from build123d import *

# Parameters (mm, degrees)
F0_W     = 450
F0_H     = 200
F1_DEPTH = 20
F3_DEPTH = 450
F4_R     = 15
F5_DEPTH = 5
F4_R_2   = 32
F4_R_3   = 30.75
F6_DEPTH = 1
F4_R_4   = 5
F7_DEPTH = 30


with BuildPart() as f1:
    # F0 (on Top) → F1 (new body)
    with BuildSketch(Plane.XY):
        Rectangle(F0_W, F0_H)
    extrude(amount=F1_DEPTH)

    # F2 (on face) → F3 (join)
    with BuildSketch(Plane.YZ.offset(225)):
        Polygon((100, 37.4977327052), (-100, 20), (100, 20), align=None)
    extrude(amount=-F3_DEPTH)

    # F4 (on face) → F5 (join)
    with BuildSketch(Plane(origin=(0, -2.4960941261, 28.5304864135), x_dir=(1, 0, 0), z_dir=(0, -0.0871557427, 0.9961946981))):
        with Locations((17.8897663927, 19.1961097517)):
            Circle(F4_R)
        with Locations((33.6060567503, -14.8038902483)):
            Circle(F4_R)
        with Locations((51.8897663927, 37.2408752097)):
            Circle(F4_R)
        with Locations((67.6060567503, 3.2408752097)):
            Circle(F4_R)
        with Locations((85.8897663927, 48.6903541087)):
            Circle(F4_R)
        with Locations((101.6060567503, 14.6903541087)):
            Circle(F4_R)
        with Locations((119.8897663927, 57.0196919143)):
            Circle(F4_R)
        with Locations((135.6060567503, 23.0196919143)):
            Circle(F4_R)
    extrude(amount=F5_DEPTH)

    # F4 (on face) → F6 (join)
    with BuildSketch(Plane(origin=(0, -2.4960941261, 28.5304864135), x_dir=(1, 0, 0), z_dir=(0, -0.0871557427, 0.9961946981))):
        with Locations((-125, 0)):
            Circle(F4_R_2)
        with Locations((-125, 0)):
            Circle(F4_R_3, mode=Mode.SUBTRACT)
    extrude(amount=F6_DEPTH)

    # F4 (on face) → F7 (join)
    with BuildSketch(Plane(origin=(0, -2.4960941261, 28.5304864135), x_dir=(1, 0, 0), z_dir=(0, -0.0871557427, 0.9961946981))):
        with Locations((-125, 0)):
            Circle(F4_R_4)
    extrude(amount=F7_DEPTH)


solid = f1.part
For this review, take the finished solid that the model builds, in its own axes (mm). A direction names the side the tool comes from. Coordinates: 2 decimals unless noted, no trailing zeros. Order: outer loops, then holes, each group sorted by start corner. A loop starts at its lowest first (then second) coordinate and runs counter-clockwise, first axis right, second up. Notation, with made-up numbers: (-11.5, 85) - (12.5, 85) arc R11 cw to (12.5, 101) - close; hole circle Ø5 at (16, 14.5). An arc over 180 degrees is marked (long way). Answer as CSV lines item,"result". Start each with the question number.
1) Add section D-D (x = -100). State the section outline as (y, z) points, then the cut area to 3 significant figures.
2) Insertion check: P1, Ø12, axis at x = -103.5, y = 75.5, coming from the +Z side; P2, Ø10, axis at x = 75.5, y = -39.5, coming from the +Z side; P3, Ø2, axis at x = 102.5, y = -22, coming from the +Z side. Each pin has a flat end and moves straight along its axis. Give the tip position at first contact, or say it passes through.
3) Machinability: for faces 5 (the flat face through (85.68, 45.782, 37.773)), 6 (the flat face through (101.4, 11.91, 34.81)), which of the approach directions +Z, -Z, +X, -X, +Y, -Y give a long, thin tool a straight path to every point of the face, cutting with its end or side? Answer none if there is none.
4) Add section A-A (x = -149.5). State the section outline as (y, z) points.
5) Add section B-B (y = -71). State the section outline as (x, z) points, then the cut area to 3 significant figures.
6) Draft analysis for pull direction Z (two halves, no side actions). For faces 1 (the flat face through (-3, -100, 10)), 2 (the cylindrical face through (-95.67, 6.66, 29.83)), 3 (the flat face through (-125.07, -5.041, 58.422)), 4 (the cylindrical face through (31.746, 10.689, 32.158)), state which applies: +Z half, -Z half, draft (parallel to the pull), parting line (faces both ways), or undercut.
7) Add section C-C (x = -20.5). State the section outline as (y, z) points.
8) To check wall thickness, follow line 1 along Z through (x, y) = (177.5, 30.5); line 2 along Z through (x, y) = (16.5, -6). State the ranges of each line that lie inside material, in increasing order. Write a range as [from, to].
Result:
1,outline,"(-100, 0) - (100, 0) - (100, 37.5) - (17.4, 30.27) - (17.32, 31.27) - (15.25, 31.09) - (15.34, 30.09) - (-20.33, 26.97) - (-20.42, 27.97) - (-22.48, 27.79) - (-22.4, 26.79) - (-100, 20) - close"
1,area,"5,750 mm^2"
2,P1,"z = 35.88"
2,P2,"z = 25.73"
2,P3,"z = 26.91"
3,face 5,"+Z, +X, -X, -Y"
3,face 6,"+Z, +X, -Y"
4,outline,"(-100, 0) - (100, 0) - (100, 37.5) - (18.01, 30.32) - (17.92, 31.32) - (15.93, 31.15) - (16.02, 30.15) - (-21.01, 26.91) - (-21.1, 27.91) - (-23.09, 27.73) - (-23, 26.74) - (-100, 20) - close"
5,outline,"(-225, 0) - (225, 0) - (225, 22.54) - (-225, 22.54) - close"
5,area,"10,100 mm^2"
6,face 1,"draft"
6,face 2,"undercut"
6,face 3,"+Z half"
6,face 4,"undercut"
7,outline,"(-100, 0) - (100, 0) - (100, 37.5) - (-100, 20) - close"
8,line 1,"[0, 31.42]"
8,line 2,"[0, 28.22]"
